```python
from build123d import *

# Parameters (mm, degrees)
F1_DEPTH = 3.81
F2_DEPTH = 228.6
F3_W     = 55
F3_H     = 220
F4_DEPTH = 25.4
F5_W     = 55
F5_H     = 220
F7_DEPTH = 228.6


with BuildPart() as f1:
    # F0 (on Top) → F1 (new body)
    with BuildSketch(Plane.XY):
        Polygon((-60.0453081081, 159.1941417708), (-56.19, 163.0041417708), (-60, 163.0041417708), (-103.7388, 119.8241417708), (-103.7388, 116.0141417708), align=None)
        Polygon((60.0809994569, 159.1941417708), (56.19, 163.0041417708), (-56.19, 163.0041417708), (-60.0453081081, 159.1941417708), (-3.8048, 159.1941417708), (0.0052, 159.1941417708), align=None)
        Polygon((-3.8048, 159.1941417708), (-60.0453081081, 159.1941417708), (-103.7388, 116.0141417708), (-103.7388, -116.4451715096), (-61.7023795136, -157.6065141999), (-3.8048, -157.4549383449), align=None)
        Polygon((0.0052, -157.4449637654), (0.0052, 159.1941417708), (-3.8048, 159.1941417708), (-3.8048, -157.4549383449), align=None)
        Polygon((103.7388, -116.3658582292), (103.7388, 116.4451715096), (60.0809994569, 159.1941417708), (0.0052, 159.1941417708), (0.0052, -157.4449637654), (61.9519895189, -157.2827870792), align=None)
        Polygon((103.7388, 119.8241417708), (60, 163.0041417708), (56.19, 163.0041417708), (60.0809994569, 159.1941417708), (103.7388, 116.4451715096), align=None)
        Polygon((103.7388, -120.1758582292), (103.7388, -116.3658582292), (61.9519895189, -157.2827870792), (56.1090005431, -163.0041417708), (60, -163.0041417708), align=None)
        Polygon((56.1090005431, -163.0041417708), (61.9519895189, -157.2827870792), (0.0052, -157.4449637654), (-3.8048, -157.4549383449), (-61.7023795136, -157.6065141999), (-56.19, -163.0041417708), align=None)
        Polygon((-61.7023795136, -157.6065141999), (-103.7388, -116.4451715096), (-103.7388, -120.1758582292), (-60, -163.0041417708), (-56.19, -163.0041417708), align=None)
    extrude(amount=-F1_DEPTH)

    # F0 (on Top) → F2 (join)
    with BuildSketch(Plane.XY):
        Polygon((60.0809994569, 159.1941417708), (56.19, 163.0041417708), (-56.19, 163.0041417708), (-60.0453081081, 159.1941417708), (-3.8048, 159.1941417708), (0.0052, 159.1941417708), align=None)
        Polygon((103.7388, 119.8241417708), (60, 163.0041417708), (56.19, 163.0041417708), (60.0809994569, 159.1941417708), (103.7388, 116.4451715096), align=None)
        Polygon((-60.0453081081, 159.1941417708), (-56.19, 163.0041417708), (-60, 163.0041417708), (-103.7388, 119.8241417708), (-103.7388, 116.0141417708), align=None)
        Polygon((56.1090005431, -163.0041417708), (61.9519895189, -157.2827870792), (0.0052, -157.4449637654), (-3.8048, -157.4549383449), (-61.7023795136, -157.6065141999), (-56.19, -163.0041417708), align=None)
        Polygon((-61.7023795136, -157.6065141999), (-103.7388, -116.4451715096), (-103.7388, -120.1758582292), (-60, -163.0041417708), (-56.19, -163.0041417708), align=None)
        Polygon((103.7388, -120.1758582292), (103.7388, -116.3658582292), (61.9519895189, -157.2827870792), (56.1090005431, -163.0041417708), (60, -163.0041417708), align=None)
        Polygon((0.0052, -157.4449637654), (0.0052, 159.1941417708), (-3.8048, 159.1941417708), (-3.8048, -157.4549383449), align=None)
    extrude(amount=F2_DEPTH)

    # F3 (on face) → F4 (cut)
    with BuildSketch(Plane.XZ.offset(163.0041417708)):
        with Locations((27.5, 114.3)):
            Rectangle(F3_W, F3_H)
        with Locations((-27.5, 114.3)):
            Rectangle(F3_W, F3_H)
    extrude(amount=-F4_DEPTH, mode=Mode.SUBTRACT)

    # F5 (on Front) → F7 (cut)
    with BuildSketch(Plane.XZ):
        with Locations((27.5, 116.84)):
            Rectangle(F5_W, F5_H)
        with Locations((-27.5, 116.84)):
            Rectangle(F5_W, F5_H)
    extrude(amount=-F7_DEPTH, mode=Mode.SUBTRACT)


solid = f1.part
```
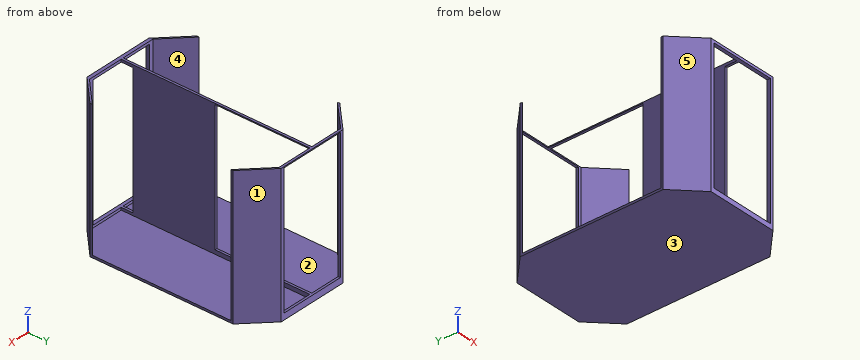
Work out the finished part from the listing and answer in its coordinate system (mm). Face numbers are marked on the shaded views. A direction names the side the tool comes from. Give positions to 0.01 mm unless a question says otherwise; leave off trailing zeros. Loops run counter-clockwise (first coordinate to the right, second up) from the corner with the lowest first, then second, coordinate; pieces in that order, holes last. Notation, with made-up numbers: M 35,48.5 L 43,48.5 A33 cw 43,84.5 Z; hole C -13.75,55 d8. An arc over 180 degrees is marked long. One line per item, written item: value. Start each with the question number.
1. Determine the mould class of the marked faces 1, 2 and 3 for opening direction X: released by +X, released by -X, zero draft, split by the parting line, or undercut.
2. Find section D-D (y = -43.5). Give the vertices of the cut face in (x, z).
3. Find section C-C (y = 92.5). Give the vertices of the cut face in (x, z), and give its area (3 significant figures).
4. Find the intervals of material crossed by probe 1 along X at (y, z) = (-128, 84); probe 2 along Z at (x, y) = (-67, -110.5); probe 3 along Y at (x, z) = (60, 216.5), in increasing order.
5. Find section A-A (z = 35). Give the vertices of the cut face in (x, y).
6. Each of these flat-tipped pins is pushed along its axis until it touches: P1, Ø4, axis at x = -2.5, z = 94, coming from the +Y side; P2, Ø1.7, axis at y = -161, z = 125, coming from the -X side; P3, Ø4.5, axis at y = -161.5, z = 161, coming from the +X side; P4, Ø10, axis at x = 8.5, z = 71, coming from the -Y side. Where does it stop, or does it pass through?
7. Find section B-B (x = -45). Give the vertices of the cut face in (y, z), and give its area (3 significant figures).
8. Which of the six approach directions +Z, -Z, +X, -X, +Y, -Y give full straight-line access (tool end or side, diameter ignored) to the marked faces 4 and 5?
Reported:
1. face 1: released by +X
1. face 2: undercut
1. face 3: zero draft
2. outline: M -103.74,-3.81 L 103.74,-3.81 L 103.74,0 L 0.01,0 L 0.01,228.6 L -3.8,228.6 L -3.8,0 L -103.74,0 Z
3. outline: M -103.74,-3.81 L 103.74,-3.81 L 103.74,0 L 0.01,0 L 0.01,6.84 L -3.8,6.84 L -3.8,0 L -103.74,0 Z; M -3.8,226.84 L 0.01,226.84 L 0.01,228.6 L -3.8,228.6 Z
3. area: 823 mm²
4. probe 1: x = -95.75 to -91.94, -3.8 to 0.01, 91.86 to 95.75
4. probe 2: z = -3.81 to 0
4. probe 3: y = -163 to -157.29, 159.19 to 163
5. outline: M -103.74,-120.18 L -60,-163 L -55,-163 L -55,-157.59 L -61.7,-157.61 L -103.74,-116.45 Z; M -103.74,116.01 L -60.05,159.19 L -55,159.19 L -55,163 L -60,163 L -103.74,119.82 Z; M -3.8,-137.6 L 0.01,-137.6 L 0.01,0 L -3.8,0 Z; M 55,-163 L 60,-163 L 103.74,-120.18 L 103.74,-116.37 L 61.95,-157.28 L 55,-157.3 Z; M 55,159.19 L 60.08,159.19 L 103.74,116.45 L 103.74,119.82 L 60,163 L 55,163 Z
6. P1: stops at y = 0
6. P2: stops at x = -62.91
6. P3: stops at x = 63.83
6. P4: passes through
7. outline: M -163,-3.81 L 163,-3.81 L 163,6.84 L 159.19,6.84 L 159.19,0 L -157.56,0 L -157.56,4.3 L -163,4.3 Z; M -163,224.3 L -157.56,224.3 L -157.56,228.6 L -163,228.6 Z; M 159.19,226.84 L 163,226.84 L 163,228.6 L 159.19,228.6 Z
7. area: 1,320 mm²
8. face 4: +Z
8. face 5: +Z, -Z, -X, -Y
